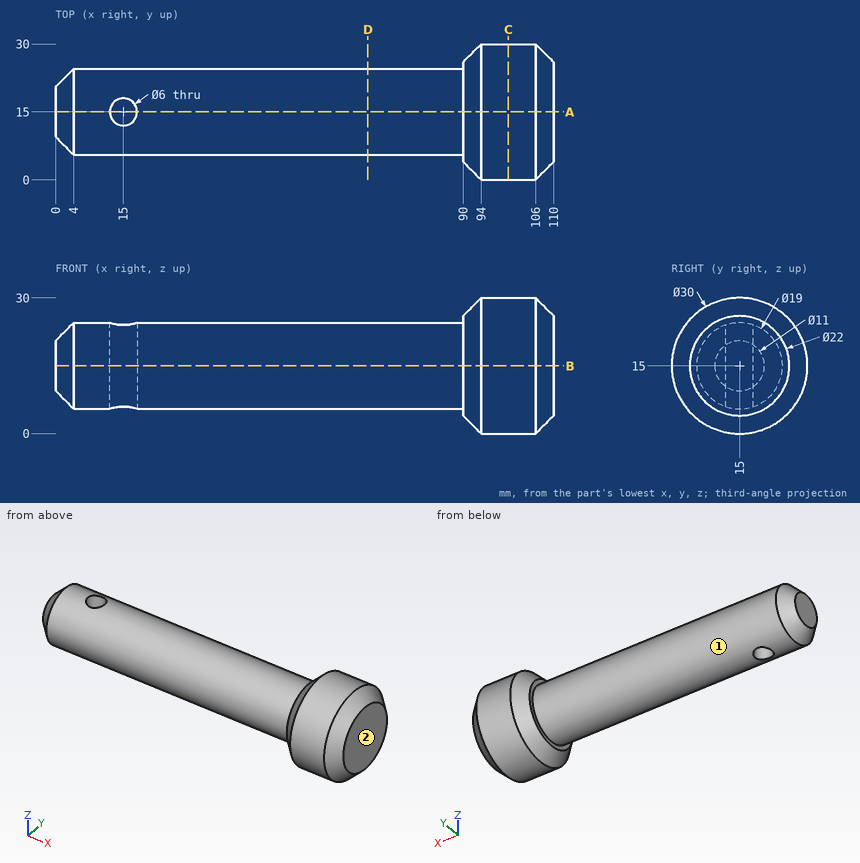
For this review, use the dimensioned drawing (mm, ordinates from the lowest corner) and the shaded views. A direction names the side the tool comes from. Give positions to 0.01 mm unless a question says otherwise; leave off trailing zeros. Loops run counter-clockwise (first coordinate to the right, second up) from the corner with the lowest first, then second, coordinate; pieces in that order, holes last. Notation, with made-up numbers: (-28, 58) - (17, 58) arc R17 cw to (17, 84) - close; hole circle Ø1 at (45.25, 10). An arc over 180 degrees is marked (long way). Write each question's results on one line, items separated by ' | '.
(1) Take a section at A-A (y = 15). Give the boundary of the cut face in (x, z), then the cut area to 3 significant figures.
Conclusion:
outline: (0, 9.5) - (4, 5.5) - (12, 5.5) - (12, 24.5) - (4, 24.5) - (0, 20.5) - close; (18, 5.5) - (90, 5.5) - (90, 4) - (94, 0) - (106, 0) - (110, 4) - (110, 26) - (106, 30) - (94, 30) - (90, 26) - (90, 24.5) - (18, 24.5) - close | area: 2,150 mm^2
(2) Take a section at C-C (x = 100). Give the boundary of the cut face in (y, z), then the cut area to 3 significant figures.
Conclusion:
outline: circle Ø30 at (15, 15) | area: 707 mm^2
(3) Take a section at B-B (z = 15). Give the boundary of the cut face in (x, y).
Conclusion:
outline: (0, 9.5) - (4, 5.5) - (90, 5.5) - (90, 4) - (94, 0) - (106, 0) - (110, 4) - (110, 26) - (106, 30) - (94, 30) - (90, 26) - (90, 24.5) - (4, 24.5) - (0, 20.5) - close; hole circle Ø6 at (15, 15)
(4) Take a section at D-D (x = 69). Give the boundary of the cut face in (y, z), then the cut area to 3 significant figures.
Conclusion:
outline: circle Ø19 at (15, 15) | area: 284 mm^2
(5) For pin 1 Ø12 at (y, z) = (3.5, 25.5) entering from -X; pin 2 Ø1 at (x, z) = (64, 7) entering from -Y; pin 3 Ø8 at (x, y) = (26, 18.5) entering from +Z, all flat-tipped, find the tip position at first contact; note any pin that passes through.
Conclusion:
pin 1: x = 90 | pin 2: y = 9.17 | pin 3: z = 24.5
(6) For the marked faces 1 and 2, list the 3-axis set-ups (+Z, -Z, +X, -X, +Y, -Y) from which the entire face can be reached by the end or side of a thin tool; tool diameter is ignored.
Conclusion:
face 1: -X | face 2: +Z, -Z, +X, +Y, -Y
(7) For line 1 along X through (y, z) = (15, 14.25); line 2 along Y through (x, z) = (15, 13); line 3 along Y through (x, z) = (57, 22.75), list the stretches that pass through material, from the lowest coordinate up.
Conclusion:
line 1: 0 to 12, 18 to 110 | line 2: 5.71 to 12, 18 to 24.29 | line 3: 9.51 to 20.49
